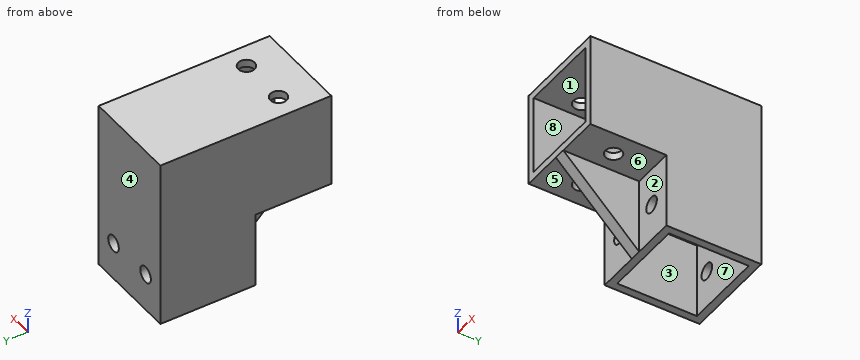
from build123d import *

# Parameters (mm, degrees)
SKETCH_W        = 45
SKETCH_H        = 25
PAD_DEPTH       = 12.5
SKETCH001_W     = 25
SKETCH001_H     = 25
PAD001_DEPTH    = 20
PAD002_DEPTH    = 1.5
SKETCH005_W     = 21
SKETCH005_H     = 21
POCKET_DEPTH    = 43
SKETCH006_W     = 21
SKETCH006_H     = 21
POCKET001_DEPTH = 20
SKETCH007_R     = 2.15
POCKET002_DEPTH = 45.001
SKETCH008_R     = 2.15
POCKET003_DEPTH = 45.001


with BuildPart() as part:
    # Sketch → Pad (new body, symmetric)
    with BuildSketch(Plane.YZ):
        with Locations((2.5, 12.5)):
            Rectangle(SKETCH_W, SKETCH_H)
    extrude(amount=PAD_DEPTH, both=True)

    # Sketch001 (on Face3 of Pad) → Pad001 (join)
    with BuildSketch(Plane.YX):
        with Locations((12.5, 0)):
            Rectangle(SKETCH001_W, SKETCH001_H)
    extrude(amount=PAD001_DEPTH)

    # Sketch004 → Pad002 (join, symmetric)
    with BuildSketch(Plane.YZ):
        Polygon((-20, 0), (0, 0), (0, -20), align=None)
    extrude(amount=PAD002_DEPTH, both=True)

    # Sketch005 (on Face2 of Pad002) → Pocket (cut)
    with BuildSketch(Plane(origin=(0, -20, 0), x_dir=(0, 0, -1), z_dir=(0, -1, 0))):
        with Locations((-12.5, 0)):
            Rectangle(SKETCH005_W, SKETCH005_H)
    extrude(amount=-POCKET_DEPTH, mode=Mode.SUBTRACT)

    # Sketch006 (on Face13 of Pocket) → Pocket001 (cut)
    with BuildSketch(Plane.YX.offset(20)):
        with Locations((12.5, 0)):
            Rectangle(SKETCH006_W, SKETCH006_H)
    extrude(amount=-POCKET001_DEPTH, mode=Mode.SUBTRACT)

    # Sketch007 (on Face3 of Pocket001) → Pocket002 (cut, through all)
    with BuildSketch(Plane.ZX.offset(25)):
        with Locations((-10, 6.5)):
            Circle(SKETCH007_R)
        with Locations((-10, -6.5)):
            Circle(SKETCH007_R)
    extrude(amount=-POCKET002_DEPTH, mode=Mode.SUBTRACT)

    # Sketch008 (on Face1 of Pocket002) → Pocket003 (cut, through all)
    with BuildSketch(Plane(origin=(0, 0, 25), x_dir=(0, -1, 0), z_dir=(0, 0, 1))):
        with Locations((10, 6.5)):
            Circle(SKETCH008_R)
        with Locations((10, -6.5)):
            Circle(SKETCH008_R)
    extrude(amount=-POCKET003_DEPTH, mode=Mode.SUBTRACT)


solid = part.part
CAD build for the part. Positions are in the model's coordinates, mm. Face numbers are marked on the shaded views. A direction names the side the tool comes from. Coordinates: 2 decimals unless noted, no trailing zeros. Loops run counter-clockwise (first coordinate to the right, second up) from the corner with the lowest first, then second, coordinate; pieces in that order, holes last. Notation, with made-up numbers: (-26.5, 55) - (23.5, 55) arc R15 cw to (23.5, 59) - close; hole circle Ø10 at (78.25, 26.5). An arc over 180 degrees is marked (long way). Use one line per item in the form item = value. Start each with the question number.
1) Band-saw the part on A-A (z = -10). Give the cut face in (x, y), and give its area (3 significant figures).
2) Flat gauge pins, fed straight in: pin 1 (5.5 mm diameter, centred on x = 6.5, z = -10, fed in from +Y); pin 2 (3.5 mm diameter, centred on x = -8.5, z = -6, fed in from -Y); pin 3 (9 mm diameter, centred on x = -9.5, y = -6, fed in from -Z); pin 4 (8 mm diameter, centred on x = 1, z = -15, fed in from -Y). Where does each tip first touch, or does it go through?
3) Band-saw the part on B-B (y = 9.5). Give the cut face in (x, z), and give its area (3 significant figures).
4) Two-plate mould, pull along Z, no slides. Class the marked faces 6, 7 and 8: +Z half, -Z half, draft (parallel to the pull), parting line (faces both ways), or undercut.
5) Drill centre lines: L1, parallel to X at y = -10, z = 24.05; L2, parallel to X at y = 8, z = -12; L3, parallel to Z at x = 9.75, y = -17. Where is each one in solid material? Low to high. Write a range as from..to.
6) Tool access for the marked faces 1, 2, 3, 4 and 5: list every direction of +Z, -Z, +X, -X, +Y, -Y with a clear straight run to the whole face (end or side of a thin tool).
7) Band-saw the part on C-C (x = 6.5). State how many separate pieces and enclosed holes the cut face has, and give its area (3 significant figures).
Check values:
q1.outline = (-12.5, 0) - (-8.65, 0) - (-8.65, 2) - (-10.5, 2) - (-10.5, 23) - (-8.65, 23) - (-8.65, 25) - (-12.5, 25) - close; (-4.35, 0) - (-1.5, 0) - (-1.5, -10) - (1.5, -10) - (1.5, 0) - (4.35, 0) - (4.35, 2) - (-4.35, 2) - close; (-4.35, 23) - (4.35, 23) - (4.35, 25) - (-4.35, 25) - close; (8.65, 0) - (12.5, 0) - (12.5, 25) - (8.65, 25) - (8.65, 23) - (10.5, 23) - (10.5, 2) - (8.65, 2) - close
q1.area = 180 mm2
q2.pin_1 = 25
q2.pin_2 = 0
q2.pin_3 = 0
q2.pin_4 = -9
q3.outline = (-12.5, -20) - (-10.5, -20) - (-10.5, 0) - (10.5, 0) - (10.5, -20) - (12.5, -20) - (12.5, 25) - (-12.5, 25) - close; hole (-10.5, 2) - (10.5, 2) - (10.5, 23) - (-10.5, 23) - close
q3.area = 264 mm2
q4.face_6 = -Z half
q4.face_7 = draft
q4.face_8 = undercut
q5.L1 = -12.5..-8.65, -4.35..4.35, 8.65..12.5
q5.L2 = -12.5..-10.5, 10.5..12.5
q5.L3 = 0..2, 23..25
q6.face_1 = -Y
q6.face_2 = -Z, +X, -Y
q6.face_3 = -Z
q6.face_4 = +Z, -Z, +X, -X, +Y
q6.face_5 = -Z, -X, -Y
q7.separate_pieces = 5
q7.enclosed_holes = 0
q7.area = 268 mm2
